Study the drawing (mm; zero at the part's minimum x, y, z) and answer. A direction names the side the tool comes from. Coordinates: 2 decimals unless noted, no trailing zeros. Order: outer loops, then holes, each group sorted by start corner. A loop starts at its lowest first (then second) coordinate and runs counter-clockwise, first axis right, second up. Notation, with made-up numbers: (27, -7) -> (47, -7) arc R33 ccw to (47, 22) -> close; hole circle Ø3 at (56.5, 49). An arc over 180 degrees is marked (long way). One line per question, with ' | ' between items.
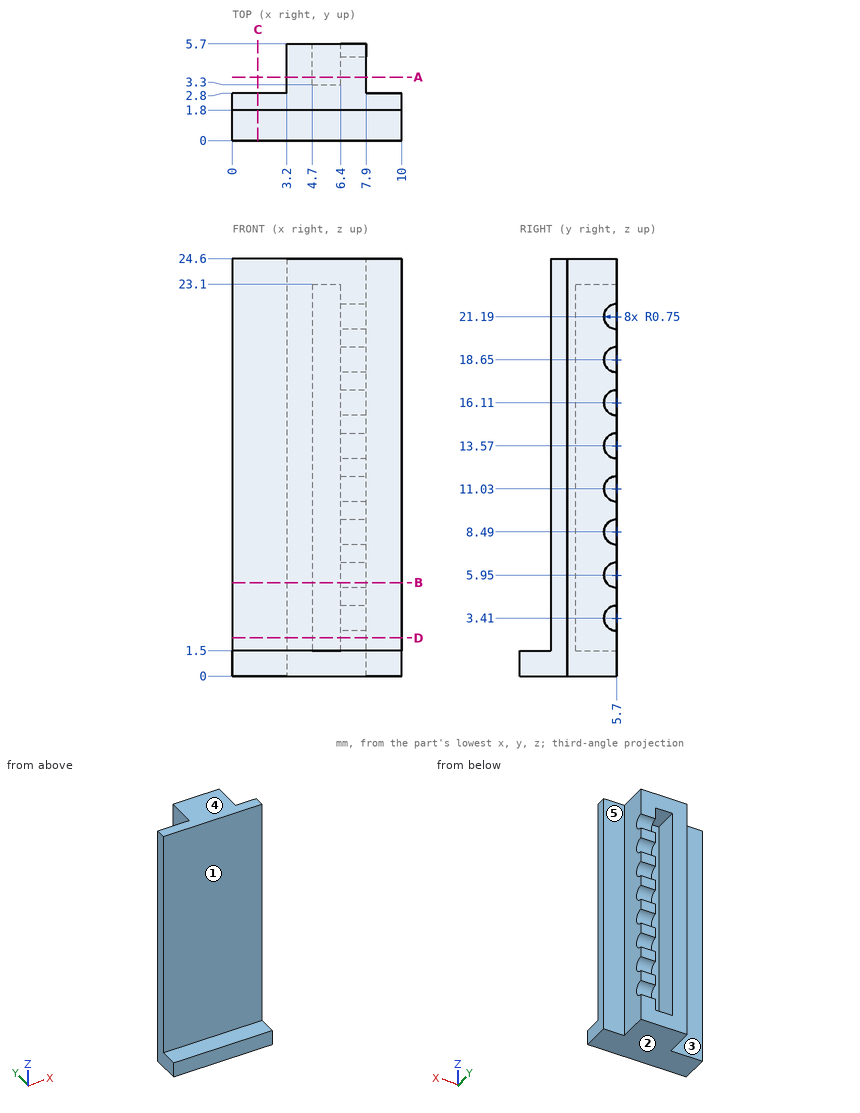
Item 1: Find the intervals of material crossed by L1, parallel to Z at x = 5.5, y = 4.7; L2, parallel to X at y = 5.15, z = 4.5; L3, parallel to Y at x = 9, z = 20, in increasing order.
Computed values:
L1: z = 0 to 1.5, 23.1 to 24.6 | L2: x = 3.2 to 4.7, 6.4 to 7.9 | L3: y = 1.8 to 2.8
Item 2: Each of these flat-tipped pins is pushed along its axis until it touches: pin 1 Ø2.5 at (y, z) = (4.5, 13) entering from -X; pin 2 Ø0.9 at (y, z) = (3.5, 9) entering from +X; pin 3 Ø1.7 at (x, z) = (9.5, 11.5) entering from +Y. Where does it stop, or does it pass through?
Computed values:
pin 1: stops at x = 3.2 | pin 2: stops at x = 7.9 | pin 3: stops at y = 2.8
Item 3: Section D-D, the plane z = 2.25 is taken. Give the vertices of the cut face in (x, y).
Computed values:
outline: (0, 1.8) -> (10, 1.8) -> (10, 2.8) -> (7.9, 2.8) -> (7.9, 5.7) -> (6.4, 5.7) -> (6.4, 3.3) -> (4.7, 3.3) -> (4.7, 5.7) -> (3.2, 5.7) -> (3.2, 2.8) -> (0, 2.8) -> close
Item 4: Section A-A, the plane y = 3.75 is taken. Give the vertices of the cut face in (x, z).
Computed values:
outline: (3.2, 0) -> (7.9, 0) -> (7.9, 24.6) -> (3.2, 24.6) -> close; hole (4.7, 1.5) -> (6.4, 1.5) -> (6.4, 23.1) -> (4.7, 23.1) -> close
Item 5: For the marked faces 1, 2, 3, 4 and 5, determine the directions among +Z, -Z, +X, -X, +Y, -Y from which every point of the face is accessible in a straight line to the end or side of a thin tool.
Computed values:
face 1: +Z, +X, -X, -Y | face 2: -Z, +X, -X, +Y, -Y | face 3: +Z, -Z, -X, +Y | face 4: +Z, +X, -X, +Y, -Y | face 5: +Z, -Z, +X, +Y
Item 6: Section B-B, the plane z = 5.5 is taken. Give the vertices of the cut face in (x, y).
Computed values:
outline: (0, 1.8) -> (10, 1.8) -> (10, 2.8) -> (7.9, 2.8) -> (7.9, 5.1) -> (6.4, 5.1) -> (6.4, 3.3) -> (4.7, 3.3) -> (4.7, 5.7) -> (3.2, 5.7) -> (3.2, 2.8) -> (0, 2.8) -> close
Item 7: Section C-C, the plane x = 1.5 is taken. Give the vertices of the cut face in (y, z), plus the area to 3 significant figures.
Computed values:
outline: (0, 0) -> (2.8, 0) -> (2.8, 24.6) -> (1.8, 24.6) -> (1.8, 1.5) -> (0, 1.5) -> close | area: 27.3 mm^2
